Read the model definition and answer for the solid it produces. Units are mm, in the model's axes. A direction names the side the tool comes from. Coordinates: 2 decimals unless noted, no trailing zeros. Loops run counter-clockwise (first coordinate to the right, second up) from the corner with the lowest first, then second, coordinate; pieces in that order, holes last.
Q1. Section C-C (z = -23.25) is taken. Give the vertices of the cut face in (x, y), then the cut area to 3 significant figures.
Q2. Section A-A (y = 21.5) is taken. Give the vertices of the cut face in (x, z), then the cut area to 3 significant figures.
Q3. Flat-ended cylindrical pins translate along their axes: P1, Ø1.5, axis at x = 3, y = 21.5, coming from the -Z side; P2, Ø3, axis at y = 6.5, z = -14, coming from the -X side; P3, Ø4, axis at x = 3, y = 13.5, coming from the -Z side; P4, Ø6, axis at x = 4, y = 7.5, coming from the -Z side. Find the tip coordinate at first contact, or state that the pin passes through.
Q4. Section B-B (x = 3) is taken. Give the vertices of the cut face in (y, z).
Q5. Section D-D (x = 9.5) is taken. Give the vertices of the cut face in (y, z), then the cut area to 3 significant figures.
Q6. Which of the six approach directions +Z, -Z, +X, -X, +Y, -Y give full straight-line access (tool end or side, diameter ignored) to faces 1 (the face through (3, 18, 0)), 2 (the face through (12, 17, -11))?
Q7. Straight lines are drawn through the part: line 1 (Y direction, x = 10.1, z = -23.25); line 2 (X direction, y = 32, z = -10); line 3 (X direction, y = 21, z = 2). For each, find the intervals that lie inside material, in ascending order.
Q8. The mould has two halves that part along Y. Classify faces 3 (the face through (9.972, 29.987, -3.945)), 4 (the face through (9, 0, -7)), 5 (the face through (8, 17, -14)): pulls with the +Y half, pulls with the -Y half, needs draft (parallel to the pull), parting line crosses it, or undercut.
from build123d import *

# Parameters (mm, degrees)
ESQUISSE1_W             = 12
ESQUISSE1_H             = 35
BOSS_EXTRU_1_DEPTH      = 5
ESQUISSE2_W             = 4
ESQUISSE2_H             = 35
BOSS_EXTRU_2_DEPTH      = 27
ESQUISSE3_R             = 1.25
ENL_V_MAT_EXTRU_1_DEPTH = 33
ESQUISSE4_R             = 1.5
ENL_V_MAT_EXTRU_2_DEPTH = 5
CONG_1_R                = 2


with BuildPart() as part:
    # Esquisse1 → Boss.-Extru.1 (new body)
    with BuildSketch(Plane.XY):
        with Locations((6, 17.5)):
            Rectangle(ESQUISSE1_W, ESQUISSE1_H)
    extrude(amount=BOSS_EXTRU_1_DEPTH)

    # Esquisse2 → Boss.-Extru.2 (add)
    with BuildSketch(Plane(origin=(0, 0, 0), x_dir=(-1, 0, 0), z_dir=(0, 0, -1))):
        with Locations((-10, 17.5)):
            Rectangle(ESQUISSE2_W, ESQUISSE2_H)
    extrude(amount=BOSS_EXTRU_2_DEPTH)

    # Esquisse3 → Enlèv. mat.-Extru.1 (cut, through all)
    with BuildSketch(Plane.XY.offset(5)):
        with Locations((3, 5.5)):
            Circle(ESQUISSE3_R)
        with Locations((3, 13.5)):
            Circle(ESQUISSE3_R)
        with Locations((3, 21.5)):
            Circle(ESQUISSE3_R)
        with Locations((3, 29.5)):
            Circle(ESQUISSE3_R)
    extrude(amount=-ENL_V_MAT_EXTRU_1_DEPTH, mode=Mode.SUBTRACT)

    # Esquisse4 → Enlèv. mat.-Extru.2 (cut, through all)
    with BuildSketch(Plane.ZY.offset(-8)):
        with Locations((-23.25, 28.5)):
            Circle(ESQUISSE4_R)
        with Locations((-3.75, 28.5)):
            Circle(ESQUISSE4_R)
        with Locations((-23.25, 6.5)):
            Circle(ESQUISSE4_R)
        with Locations((-3.75, 6.5)):
            Circle(ESQUISSE4_R)
    extrude(amount=-ENL_V_MAT_EXTRU_2_DEPTH, mode=Mode.SUBTRACT)

    # Congé1
    cong_1_edges = [part.edges().sort_by_distance(p)[0] for p in [
        (8, 17.5, 0),
    ]]
    fillet(cong_1_edges, radius=CONG_1_R)


solid = part.part
Numbers:
1. outline: (8, 0) - (12, 0) - (12, 5) - (8, 5) - close; (8, 8) - (12, 8) - (12, 27) - (8, 27) - close; (8, 30) - (12, 30) - (12, 35) - (8, 35) - close
1. area: 116 mm2
2. outline: (0, 0) - (1.75, 0) - (1.75, 5) - (0, 5) - close; (4.25, 0) - (6, 0) arc R2 cw to (8, -2) - (8, -27) - (12, -27) - (12, 5) - (4.25, 5) - close
2. area: 156 mm2
3. P1: passes through
3. P2: stops at x = 8
3. P3: stops at z = 0
3. P4: stops at z = -0.27
4. outline: (0, 0) - (4.25, 0) - (4.25, 5) - (0, 5) - close; (6.75, 0) - (12.25, 0) - (12.25, 5) - (6.75, 5) - close; (14.75, 0) - (20.25, 0) - (20.25, 5) - (14.75, 5) - close; (22.75, 0) - (28.25, 0) - (28.25, 5) - (22.75, 5) - close; (30.75, 0) - (35, 0) - (35, 5) - (30.75, 5) - close
5. outline: (0, -27) - (35, -27) - (35, 5) - (0, 5) - close; hole circle Ø3 at (6.5, -23.25); hole circle Ø3 at (6.5, -3.75); hole circle Ø3 at (28.5, -23.25); hole circle Ø3 at (28.5, -3.75)
5. area: 1,090 mm2
6. face 1: -Z, -X, +Y, -Y
6. face 2: +Z, -Z, +X, +Y, -Y
7. line 1: y = 0 to 5, 8 to 27, 30 to 35
7. line 2: x = 8 to 12
7. line 3: x = 0 to 1.85, 4.15 to 12
8. face 3: undercut
8. face 4: pulls with the -Y half
8. face 5: needs draft
